Model file for the job. Use its own axes, mm. Coordinates: 2 decimals unless noted, no trailing zeros. Order: outer loops, then holes, each group sorted by start corner. A loop starts at its lowest first (then second) coordinate and runs counter-clockwise, first axis right, second up. Notation, with made-up numbers: M 52.25,58.25 L 89.25,58.25 A33 cw 89.25,96.25 Z; hole C 12,11 d3. An arc over 180 degrees is marked long. Return JSON: item names as keys, results as strings.
```python
from build123d import *

# Parameters (mm, degrees)
SKETCH_18_W          = 50
SKETCH_18_H          = 40
EXTRUDE_2_DEPTH      = 40
CUT_EXTRUDE_9_DEPTH  = 40
CUT_EXTRUDE_10_DEPTH = 40


with BuildPart() as part:
    # 草圖18 → 填料-伸長2 (new body)
    with BuildSketch(Plane(origin=(0, 0, 0), x_dir=(1, 0, 0), z_dir=(0, 1, 0))):
        Rectangle(SKETCH_18_W, SKETCH_18_H)
    extrude(amount=EXTRUDE_2_DEPTH)

    # 草圖28 → 除料-伸長9 (cut)
    with BuildSketch(Plane(origin=(15.963302752, 21.28440367, 7.981651376), x_dir=(0.818367137, -0.538104419, -0.201789157), z_dir=(0.574695771, 0.766261028, 0.287347886))):
        Polygon((-37.835466942, -4.681645888), (-25.616012434, 14.044937664), (11.042351093, -15.215349135), align=None)
    extrude(amount=CUT_EXTRUDE_9_DEPTH, mode=Mode.SUBTRACT)

    # 草圖31 → 除料-伸長10 (cut)
    with BuildSketch(Plane(origin=(6.052631579, 18.157894737, 18.157894737), x_dir=(-0.973328527, 0.162221421, 0.162221421), z_dir=(-0.229415734, -0.688247202, -0.688247202))):
        Polygon((11.355499479, 28.284271247), (-19.466570536, 35.355339059), (-19.466570536, -7.071067812), align=None)
    extrude(amount=-CUT_EXTRUDE_10_DEPTH, mode=Mode.SUBTRACT)


solid = part.part
```
Item 1: Saw through at C-C (x = 13). Write the cut outline in (y, z).
Check result:
{"outline": "M 0,-20 L 40,-20 L 40,-6 L 22,12 L 19,20 L 0,20 Z"}
Item 2: Wall check: line 1 (Y direction, x = 0, z = 9) (3 decimals); line 2 (Y direction, x = 17.5, z = -6.5); line 3 (Z direction, x = 15.5, y = 26). Give the ranges that are in metal, low to high.
Check result:
{"line 1": "y = 0 to 32.875", "line 2": "y = 0 to 39", "line 3": "z = -20 to 7.17"}
Item 3: Saw through at B-B (z = -3). Write the cut outline in (x, y), and give its area (3 significant figures).
Check result:
{"outline": "M -25,0 L 25,0 L 25,33 L 4,40 L -25,40 Z", "area": "1,930 mm2"}
Item 4: Saw through at A-A (y = 31). Write the cut outline in (x, z).
Check result:
{"outline": "M -25,-20 L 25,-20 L 25,-1 L 4,6 L -3,20 L -25,20 Z"}
